```python
from build123d import *

# Parameters (mm, degrees)
F0_W     = 50.8
F0_H     = 50.8
F1_DEPTH = 50.8
F2_W     = 28.448
F2_H     = 27.305
F3_DEPTH = 25.4
F4_R     = 15.517483
F5_DEPTH = 50.8


with BuildPart() as f1:
    # F0 (on Front) → F1 (new body)
    with BuildSketch(Plane.XZ):
        with Locations((-25.4, 25.4)):
            Rectangle(F0_W, F0_H)
    extrude(amount=F1_DEPTH)

    # F2 (on face) → F3 (join)
    with BuildSketch(Plane(origin=(-50.8, 0, 0), x_dir=(0, -1, 0), z_dir=(-1, 0, 0))):
        with Locations((14.224, 37.1475)):
            Rectangle(F2_W, F2_H)
    extrude(amount=F3_DEPTH)

    # F4 (on face) → F5 (cut)
    with BuildSketch(Plane(origin=(0, 0, 0), x_dir=(1, 0, 0), z_dir=(0, 0, -1))):
        with Locations((-25.4, 25.4)):
            Circle(F4_R)
    extrude(amount=-F5_DEPTH, mode=Mode.SUBTRACT)


solid = f1.part
```
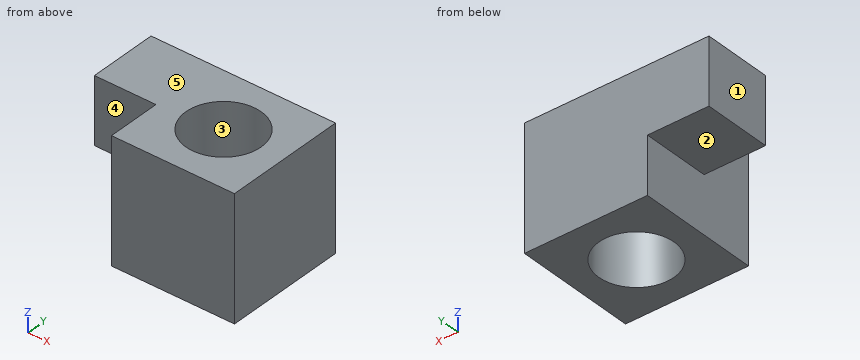
The listing builds one solid part. Answer for the finished solid, in the listing's coordinates (mm). Face numbers are marked on the shaded views. A direction names the side the tool comes from. Round coordinates to 2 decimals unless told otherwise and drop trailing zeros. Loops run counter-clockwise (first coordinate to the right, second up) from the corner with the lowest first, then second, coordinate; pieces in that order, holes last.
Q1. Section D-D, the plane y = -17 is taken. Determine the outline of the cut face in (x, z) (3 decimals).
Q2. Given pin 1 Ø2 at (x, y) = (-58.5, -27.5) entering from -Z (3 decimals); pin 2 Ø1.5 at (y, z) = (-31, 34) entering from -X; pin 3 Ø7.5 at (x, z) = (-69.5, 36.5) entering from -Y, each flat-ended and moving along its own axis, determine where each tip first touches the part or whether it passes through.
Q3. Section B-B, the plane x = -25.4 is taken. Determine the outline of the cut face in (y, z).
Q4. Section A-A, the plane y = -25.4 is taken. Determine the outline of the cut face in (x, z) (3 decimals), then the cut area to 3 significant figures.
Q5. Find the intervals of material crossed by line 1 (Y direction, x = -25, z = 7.5); line 2 (X direction, y = -25.4, z = 18.5); line 3 (X direction, y = -25, z = 24.5), in increasing order.
Q6. Section C-C, the plane z = 45.5 is taken. Determine the outline of the cut face in (x, y), then the cut area to 3 significant figures.
Q7. Which of the six approach directions +Z, -Z, +X, -X, +Y, -Y give full straight-line access (tool end or side, diameter ignored) to the marked faces 4 and 5?
Q8. For a pull along X with two mould halves and no side action, classify the marked faces 1, 2 and 3 as released by +X, released by -X, zero draft, split by the parting line, or undercut.
Completed:
1. outline: (-76.2, 23.495) - (-50.8, 23.495) - (-50.8, 0) - (-38.447, 0) - (-38.447, 50.8) - (-76.2, 50.8) - close; (-12.353, 0) - (0, 0) - (0, 50.8) - (-12.353, 50.8) - close
2. pin 1: stops at z = 23.495
2. pin 2: stops at x = -50.8
2. pin 3: stops at y = -28.45
3. outline: (-50.8, 0) - (-40.92, 0) - (-40.92, 50.8) - (-50.8, 50.8) - close; (-9.88, 0) - (0, 0) - (0, 50.8) - (-9.88, 50.8) - close
4. outline: (-76.2, 23.495) - (-50.8, 23.495) - (-50.8, 0) - (-40.917, 0) - (-40.917, 50.8) - (-76.2, 50.8) - close; (-9.883, 0) - (0, 0) - (0, 50.8) - (-9.883, 50.8) - close
4. area: 1,700 mm2
5. line 1: y = -50.8 to -40.91, -9.89 to 0
5. line 2: x = -50.8 to -40.92, -9.88 to 0
5. line 3: x = -76.2 to -40.91, -9.89 to 0
6. outline: (-76.2, -28.45) - (-50.8, -28.45) - (-50.8, -50.8) - (0, -50.8) - (0, 0) - (-76.2, 0) - close; hole circle Ø31.03 at (-25.4, -25.4)
6. area: 2,550 mm2
7. face 4: +Z, -Z, -X, -Y
7. face 5: +Z, +X, -X, +Y, -Y
8. face 1: released by -X
8. face 2: zero draft
8. face 3: undercut
